```python
from build123d import *

# Parameters (mm, degrees)
SKETCH1_R                = 42.5
SKETCH1_R_2              = 5
BOSS_EXTRUDE1_DEPTH      = 5
SKETCH2_R                = 1.2
SKETCH2_R_2              = 1.225
SKETCH2_R_3              = 5.05
SKETCH2_R_4              = 1.015
CUT_EXTRUDE1_DEPTH       = 10
SKETCH5_R                = 5
SKETCH5_R_2              = 1.015
BOSS_EXTRUDE2_DEPTH      = 6
SKETCH9_R                = 2.357259082
BOSS_EXTRUDE4_DEPTH      = 1
FILLET1_R                = 1
SKETCH10_R               = 1.5
CUT_EXTRUDE3_DEPTH       = 2.2
CUT_EXTRUDE3_DEPTH_BACK  = 16
CUT_EXTRUDE6_DEPTH       = 0.5
CUT_EXTRUDE7_DEPTH       = 10
CUT_EXTRUDE8_DEPTH       = 10
CUT_EXTRUDE8_DEPTH_BACK  = 10
CUT_EXTRUDE9_DEPTH       = 10
CUT_EXTRUDE9_DEPTH_BACK  = 10
SKETCH17_R               = 5.5
CUT_EXTRUDE10_DEPTH      = 10
CUT_EXTRUDE10_DEPTH_BACK = 10
SKETCH18_R               = 2.25
CUT_EXTRUDE11_DEPTH      = 2.2


with BuildPart() as part:
    # Sketch1 → Boss-Extrude1 (new body)
    with BuildSketch(Plane(origin=(0, 0, 0), x_dir=(1, 0, 0), z_dir=(0, 1, 0))):
        Circle(SKETCH1_R)
        with Locations((-5.00907497, -17.981343775)):
            Circle(SKETCH1_R_2, mode=Mode.SUBTRACT)
    extrude(amount=BOSS_EXTRUDE1_DEPTH)

    # Sketch2 → Cut-Extrude1 (cut)
    with BuildSketch(Plane(origin=(0, 5, 0), x_dir=(1, 0, 0), z_dir=(0, 1, 0))):
        with Locations((22.761295372, 5.470231528)):
            Circle(SKETCH2_R)
        with Locations((13.931063063, 18.812907323)):
            Circle(SKETCH2_R)
        with Locations((9.801070346, 6.486384692)):
            Circle(SKETCH2_R_2)
        with Locations((18.346179218, 12.141569425)):
            Circle(SKETCH2_R_3)
        with Locations((5.141105692, 15.974131645)):
            Circle(SKETCH2_R_4)
    extrude(amount=-CUT_EXTRUDE1_DEPTH, mode=Mode.SUBTRACT)

    # Sketch5 → Boss-Extrude2 (add)
    with BuildSketch(Plane(origin=(0, 5, 0), x_dir=(1, 0, 0), z_dir=(0, 1, 0))):
        with Locations((-10.748331153, 12.120782872)):
            Circle(SKETCH5_R)
        with Locations((-10.748331153, 12.120782872)):
            Circle(SKETCH5_R_2, mode=Mode.SUBTRACT)
    extrude(amount=BOSS_EXTRUDE2_DEPTH)

    # Sketch9 → Boss-Extrude4 (add)
    with BuildSketch(Plane.XZ):
        with Locations((5.141105692, -15.974131645)):
            Circle(SKETCH9_R)
    extrude(amount=-BOSS_EXTRUDE4_DEPTH)

    # Fillet1
    fillet1_edges = [part.edges().sort_by_distance(p)[0] for p in [
        (-42.5, 5, 0),
    ]]
    fillet(fillet1_edges, radius=FILLET1_R)

    # Sketch10 → Cut-Extrude3 (cut, two sides)
    with BuildSketch(Plane(origin=(0, 5, 0), x_dir=(1, 0, 0), z_dir=(0, 1, 0))) as cut_extrude3_sk:
        with Locations((0, 37.8)):
            Circle(SKETCH10_R)
        with Locations((-32.735760263, -18.9)):
            Circle(SKETCH10_R)
        with Locations((32.735760263, -18.9)):
            Circle(SKETCH10_R)
    extrude(amount=CUT_EXTRUDE3_DEPTH, mode=Mode.SUBTRACT)
    extrude(cut_extrude3_sk.sketch, amount=-CUT_EXTRUDE3_DEPTH_BACK, mode=Mode.SUBTRACT)

    # Sketch12 → Cut-Extrude6 (cut)
    with BuildSketch(Plane.XZ):
        with BuildLine():
            Line((-18.74897508, 25.683138694), (-31.97397508, 2.776766764))
            ThreePointArc((-31.97397508, 2.776766764), (-32.473477192, -1.017328462), (-30.143848061, -4.053360255))
            Line((-30.143848061, -4.053360255), (-11.524301879, -14.803360255))
            ThreePointArc((-11.524301879, -14.803360255), (-7.730206654, -15.302862368), (-4.694174861, -12.973233236))
            Line((-4.694174861, -12.973233236), (8.530825139, 9.933138694))
            ThreePointArc((8.530825139, 9.933138694), (2.76592503, 31.448038804), (-18.74897508, 25.683138694))
        make_face()
    extrude(amount=-CUT_EXTRUDE6_DEPTH, mode=Mode.SUBTRACT)

    # Sketch13 → Cut-Extrude7 (cut)
    with BuildSketch(Plane(origin=(0, 5, 0), x_dir=(1, 0, 0), z_dir=(0, 1, 0))):
        with BuildLine():
            Line((32.816836472, -6.07169605), (21.984996749, -21.138640776))
            ThreePointArc((21.984996749, -21.138640776), (16.391033491, -22.978825985), (12.925236211, -18.21784334))
            Line((12.925236211, -18.21784334), (12.931687147, -3.407234286))
            ThreePointArc((12.931687147, -3.407234286), (14.35531099, 0.084802692), (17.813324255, 1.589186743))
            Line((17.813324255, 1.589186743), (28.638713042, 1.845522414))
            ThreePointArc((28.638713042, 1.845522414), (33.179093412, -0.819461796), (32.816836472, -6.07169605))
        make_face()
    extrude(amount=-CUT_EXTRUDE7_DEPTH, mode=Mode.SUBTRACT)

    # Sketch15 → Cut-Extrude8 (cut, two sides)
    with BuildSketch(Plane.XZ.offset(-0.5)) as cut_extrude8_sk:
        with BuildLine():
            Line((-4.454061063, -15.186961023), (-14.190064184, -29.028285448))
            ThreePointArc((-14.190064184, -29.028285448), (-14.263329759, -31.217660805), (-12.286203391, -32.160901823))
            Line((-12.286203391, -32.160901823), (11.926297184, -28.886712635))
            ThreePointArc((11.926297184, -28.886712635), (14.476623444, -26.492368994), (13.043930349, -23.301062679))
            Line((13.043930349, -23.301062679), (-1.808225202, -14.611372289))
            ThreePointArc((-1.808225202, -14.611372289), (-3.243361659, -14.383326468), (-4.454061063, -15.186961023))
        make_face()
    extrude(amount=CUT_EXTRUDE8_DEPTH, mode=Mode.SUBTRACT)
    extrude(cut_extrude8_sk.sketch, amount=-CUT_EXTRUDE8_DEPTH_BACK, mode=Mode.SUBTRACT)

    # Sketch16 → Cut-Extrude9 (cut, two sides)
    with BuildSketch(Plane.XZ.offset(-0.5)) as cut_extrude9_sk:
        with BuildLine():
            Line((-12.984156175, 14.705600426), (-13.719701132, 11.95882482))
            ThreePointArc((-13.719701132, 11.95882482), (-13.693758532, 7.802544191), (-11.54963643, 4.241914739))
            Line((-11.54963643, 4.241914739), (-10.842839117, 3.568938111))
            ThreePointArc((-10.842839117, 3.568938111), (-9.907482144, -2.457917187), (-15.493944375, -4.905225341))
            Line((-15.493944375, -4.905225341), (-19.004093622, -4.034917019))
            ThreePointArc((-19.004093622, -4.034917019), (-20.457115896, -3.417911536), (-21.645362284, -2.3786618))
            Line((-21.645362284, -2.3786618), (-25.653320737, 2.441392154))
            ThreePointArc((-25.653320737, 2.441392154), (-26.807383132, 5.519886283), (-25.80025353, 8.649531003))
            Line((-25.80025353, 8.649531003), (-19.012059198, 17.647148968))
            ThreePointArc((-19.012059198, 17.647148968), (-14.786139745, 18.659973084), (-12.984156175, 14.705600426))
        make_face()
    extrude(amount=CUT_EXTRUDE9_DEPTH, mode=Mode.SUBTRACT)
    extrude(cut_extrude9_sk.sketch, amount=-CUT_EXTRUDE9_DEPTH_BACK, mode=Mode.SUBTRACT)

    # Sketch17 → Cut-Extrude10 (cut, two sides)
    with BuildSketch(Plane.XZ.offset(-0.5)) as cut_extrude10_sk:
        Circle(SKETCH17_R)
    extrude(amount=CUT_EXTRUDE10_DEPTH, mode=Mode.SUBTRACT)
    extrude(cut_extrude10_sk.sketch, amount=-CUT_EXTRUDE10_DEPTH_BACK, mode=Mode.SUBTRACT)

    # Sketch18 → Cut-Extrude11 (cut)
    with BuildSketch(Plane(origin=(0, 5, 0), x_dir=(1, 0, 0), z_dir=(0, 1, 0))):
        with Locations((13.931063063, 18.812907323)):
            Circle(SKETCH18_R)
        with Locations((22.761295372, 5.470231528)):
            Circle(SKETCH18_R)
    extrude(amount=-CUT_EXTRUDE11_DEPTH, mode=Mode.SUBTRACT)


solid = part.part
```
The model under review builds one solid part; all positions refer to its coordinate system, in mm. A direction names the side the tool comes from. Give positions to 0.01 mm unless a question says otherwise; leave off trailing zeros. Write each loop counter-clockwise with the first axis right and the second up, starting at its lowest first coordinate (ties: lowest second). Pieces come first, ordered by that corner, then holes. Notation, with made-up numbers: M 55.5,46 L 112.5,46 A29 cw 112.5,68 Z; hole C 27,45.5 d11. An arc over 180 degrees is marked long. Write each question's results on one line, items separated by ' | '. Start each with the question number.
1. Mouldability with a two-part tool opening along Z and no side actions: class faces 4 (the cylindrical face through (-33.727, 1.972, 25.861)), 5 (the flat face through (-10.8, 11, -13.3)), 6 (the flat face through (27.477, 2.535, 13.5)), 7 (the cylindrical face through (20.513, 3.915, -5.569)) as released by +Z, released by -Z, zero draft, split by the parting line, or undercut.
2. Insertion check: pin 1 Ø3.5 at (x, z) = (23, -6.5) entering from +Y; pin 2 Ø6 at (x, y) = (8, 3.5) entering from +Z; pin 3 Ø1 at (x, y) = (-17, 1.5) entering from -Z; pin 4 Ø9 at (x, z) = (0, 0) entering from +Y. Each pin has a flat end and moves straight along its axis. Give the tip position at first contact, or say it passes through.
3. We need section A-A (z = 0). Write out the cut boundary in (x, y), and give its area (3 significant figures).
4. For probe 1 along Z at (x, y) = (23.5, 1); probe 2 along Z at (x, y) = (-3, 1.25); probe 3 along Z at (x, y) = (21, 2.75), list the stretches that pass through material, from the lowest coordinate up. Write a range as [from, to].
5. We need section B-B (y = 7.25). Write out the cut boundary in (x, z) (3 decimals), and give its area (3 significant figures).
6. For faces 1 (the flat face through (-17.224, 2.718, -4.476)), 2 (the flat face through (-20.964, 0.246, -9.353)), 3 (the flat face through (14.9, 2.8, -17.8)), list the 3-axis set-ups (+Z, -Z, +X, -X, +Y, -Y) from which the entire face can be reached by the end or side of a thin tool; tool diameter is ignored.
Results found:
1) face 4: split by the parting line | face 5: zero draft | face 6: undercut | face 7: undercut
2) pin 1: stops at y = 5 | pin 2: stops at z = 42.2 | pin 3: stops at z = -39.17 | pin 4: passes through
3) outline: M -42.5,0 L -32.64,0 L -32.64,0.5 L -23.62,0.5 L -23.62,5 L -41.5,5 A1 ccw -42.5,4 Z; M -9.29,0.5 L -5.5,0.5 L -5.5,5 L -9.29,5 Z; M 5.5,0 L 14.27,0 L 14.27,5 L 5.5,5 Z; M 32.64,0 L 42.5,0 L 42.5,4 A1 ccw 41.5,5 L 32.64,5 Z | area: 200 mm^2
4) probe 1: z = [-35.41, -6.42], [-4.52, -1.72], [19.03, 35.41] | probe 2: z = [-42.39, -30.91], [-14.35, -4.61], [4.61, 13.4], [22.56, 42.39] | probe 3: z = [-36.95, -16.44], [-7.85, -1.66], [22.16, 36.95]
5) outline: C -10.748,-12.121 d10; hole C -10.748,-12.121 d2.03 | area: 75.3 mm^2
6) face 1: +Y, -Y | face 2: -Y | face 3: +Y
